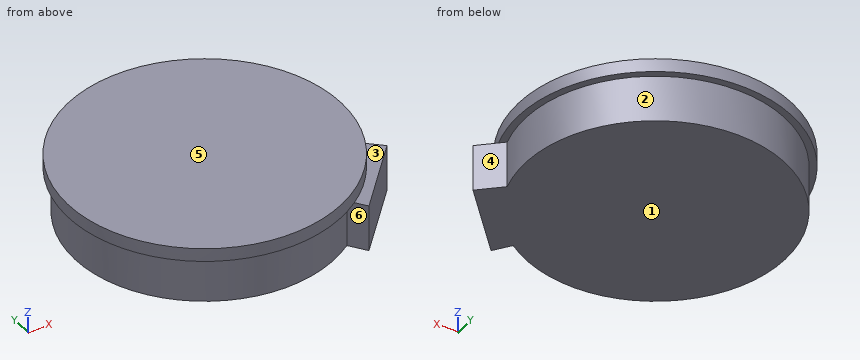
from build123d import *

# Parameters (mm, degrees)
F0_R     = 49.650765
F1_DEPTH = 17.78
F2_R     = 52.245566
F3_DEPTH = 5.08
F5_DEPTH = 17.78


with BuildPart() as f1:
    # F0 (on Top) → F1 (new body)
    with BuildSketch(Plane.XY):
        Circle(F0_R)
    extrude(amount=F1_DEPTH)

    # F2 (on face) → F3 (join)
    with BuildSketch(Plane.XY.offset(17.78)):
        Circle(F2_R)
    extrude(amount=F3_DEPTH)

    # F4 (on Top) → F5 (join)
    with BuildSketch(Plane.XY):
        Polygon((46.185026, -12.667159), (24.616234, -34.781907), (33.415832, -46.560664), (55.981882, -21.482732), align=None)
    extrude(amount=F5_DEPTH)


solid = f1.part
Can you work these out from the model? Positions are in its coordinate system, mm. Face numbers are marked on the shaded views. A direction names the side the tool comes from. Round coordinates to 2 decimals unless told otherwise and drop trailing zeros. Write each loop counter-clockwise with the first axis right and the second up, starting at its lowest first coordinate (ties: lowest second). Pieces come first, ordered by that corner, then holes. Notation, with made-up numbers: (3.5, 31.5) -> (49.5, 31.5) arc R8 cw to (49.5, 39.5) -> close; hole circle Ø4 at (33.25, 3). An arc over 180 degrees is marked (long way). Use one line per item in the form item = value. Start each with the question number.
Q1. Imagine slicing it at A-A (x = 0). Please give me the cut outline in (y, z), then the cut area to 3 significant figures.
Q2. Which directions (+Z, -Z, +X, -X, +Y, -Y) give clear straight access to the entire face, cutting with the end or side of a thin tool? Please do the marked faces 1, 2 and 3.
Q3. If I drill on probe 1 along Y at (x, z) = (1, 10.5); probe 2 along Z at (x, y) = (46, -29); probe 3 along X at (y, z) = (32.5, 19.75), over which ranges is the centre line in solid material (lowest first)? Write a range as [from, to].
Q4. Imagine slicing it at C-C (z = 12). Please give me the cut outline in (x, y), then the cut area to 3 significant figures.
Q5. We'd pull the mould along X, two halves only. Please class the marked faces 4, 5 and 6: +X half, -X half, draft (parallel to the pull), parting line (faces both ways), or undercut.
Q6. I'm going to push flat-ended pins straight in: P1, Ø12, axis at y = -27, z = 12.5, coming from the -X side; P2, Ø1, axis at x = -37, z = 17, coming from the +Y side; P3, Ø6, axis at x = 36, z = 8, coming from the +Y side. Where does each tip first touch, or does it pass through?
Worked out:
q1.outline = (-52.25, 17.78) -> (-49.65, 17.78) -> (-49.65, 0) -> (49.65, 0) -> (49.65, 17.78) -> (52.25, 17.78) -> (52.25, 22.86) -> (-52.25, 22.86) -> close
q1.area = 2,300 mm^2
q2.face_1 = -Z, +X, -X, +Y, -Y
q2.face_2 = -Z
q2.face_3 = +Z, +X, -Y
q3.probe_1 = [-49.64, 49.64]
q3.probe_2 = [0, 17.78]
q3.probe_3 = [-40.91, 40.91]
q4.outline = (28.83, -40.42) -> (33.42, -46.56) -> (55.98, -21.48) -> (47.64, -13.98) arc R49.65 ccw (long way) to start
q4.area = 7,990 mm^2
q5.face_4 = +X half
q5.face_5 = draft
q5.face_6 = undercut
q6.P1 = -46.33
q6.P2 = 33.66
q6.P3 = 37.1
